from build123d import *

# Parameters (mm, degrees)
SKETCH1_R           = 12
SKETCH1_R_2         = 1.05
BOSS_EXTRUDE1_DEPTH = 9.1
HOLE2_D             = 7
HOLE2_DEPTH         = 12
HOLE2_CBORE_D       = 9
HOLE2_CBORE_DEPTH   = 3.9
SKETCH8_R           = 2.15
CUT_EXTRUDE1_DEPTH  = 6.2
FILLET1_R           = 1


with BuildPart() as part:
    # Sketch1 → Boss-Extrude1 (new body)
    with BuildSketch(Plane.XY):
        Circle(SKETCH1_R)
        with Locations((0, 8)):
            Circle(SKETCH1_R_2, mode=Mode.SUBTRACT)
        with Locations((8, 0)):
            Circle(SKETCH1_R_2, mode=Mode.SUBTRACT)
        with Locations((0, -8)):
            Circle(SKETCH1_R_2, mode=Mode.SUBTRACT)
    extrude(amount=BOSS_EXTRUDE1_DEPTH)

    # Hole2
    with Locations(Plane.XY.offset(9.1)):
        with Locations((-6, 0)):
            CounterBoreHole(HOLE2_D / 2, HOLE2_CBORE_D / 2, HOLE2_CBORE_DEPTH, depth=HOLE2_DEPTH)

    # Sketch8 → Cut-Extrude1 (cut)
    with BuildSketch(Plane(origin=(0, 0, 0), x_dir=(-1, 0, 0), z_dir=(0, 0, -1))):
        with Locations((0, 8)):
            Circle(SKETCH8_R)
        with Locations((0, -8)):
            Circle(SKETCH8_R)
        with Locations((-8, 0)):
            Circle(SKETCH8_R)
    extrude(amount=-CUT_EXTRUDE1_DEPTH, mode=Mode.SUBTRACT)

    # Fillet1
    fillet1_edges = [part.edges().sort_by_distance(p)[0] for p in [
        (-12, 0, 0),
        (-2.5, 0, 0),
        (-2.5, 0, 5.2),
        (-12, 0, 9.1),
    ]]
    fillet(fillet1_edges, radius=FILLET1_R - 0.0001)  # a hair under: the kernel refuses the full size


solid = part.part
Can you work these out from the model? Positions are in its coordinate system, mm. A direction names the side the tool comes from. Coordinates: 2 decimals unless noted, no trailing zeros. Order: outer loops, then holes, each group sorted by start corner. A loop starts at its lowest first (then second) coordinate and runs counter-clockwise, first axis right, second up. Notation, with made-up numbers: (84, 2) - (109, 2) arc R23 cw to (109, 31) - close; hole circle Ø11 at (4, 23.5). An arc over 180 degrees is marked (long way). Answer as a JSON object with one key per item and string values. Group by question number.
Q1. We'd pull the mould along X, two halves only. Please class faces 4 (the face through (-11.99, 0.53, 4.5)), 5 (the face through (0, 0, 0)), 6 (the face through (7, 1, 6.2)): +X half, -X half, draft (parallel to the pull), parting line (faces both ways), or undercut.
Q2. Imagine slicing it at B-B (x = 0). Please give me the cut outline in (y, z).
Q3. I need wall thicknesses on line 1 (Y direction, x = 0, z = 2.75); line 2 (Y direction, x = 0, z = 6.85); line 3 (X direction, y = -0.25, z = 2). Which ranges of each line are inside material? Lowest first, please. Write a range as from..to.
Q4. On a 3-axis mill with a long thin cutter (end or side, diameter ignored), from which of +Z, -Z, +X, -X, +Y, -Y can I reach the whole of each face in a straight line? I mean faces 1 (the face through (-10.496, 0.198, 7.177)), 2 (the face through (2, 0, 9.1)), 3 (the face through (-1, 9, 6.2)). Say none if no direction works.
Q5. Imagine slicing it at A-A (y = 0). Give the number of separate pieces and of enclosed holes in the cut face, and give its area (3 significant figures).
Q6. Will these pins go through, and if not, where does the flat tip stop? P1, Ø2, axis at x = 0.5, y = 7, coming from the -Z side; P2, Ø1.5, axis at x = -4.5, z = 2.5, coming from the +Y side; P3, Ø1.5, axis at x = 9, y = 8.5, coming from the +Z side.
Q7. Imagine slicing it at C-C (z = 2.5). Please give me the cut outline in (x, y).
Determined:
{
 "1": {"face 4": "parting line", "face 5": "draft", "face 6": "undercut"},
 "2": {"outline": "(-12, 1) arc R1 ccw to (-11, 0) - (-10.15, 0) - (-10.15, 6.2) - (-9.05, 6.2) - (-9.05, 9.1) - (-11, 9.1) arc R1 ccw to (-12, 8.1) - close; (-6.95, 6.2) - (-5.85, 6.2) - (-5.85, 0) - (5.85, 0) - (5.85, 6.2) - (6.95, 6.2) - (6.95, 9.1) - (-6.95, 9.1) - close; (9.05, 6.2) - (10.15, 6.2) - (10.15, 0) - (11, 0) arc R1 ccw to (12, 1) - (12, 8.1) arc R1 ccw to (11, 9.1) - (9.05, 9.1) - close"},
 "3": {"line 1": "y = -12..-10.15, -5.85..5.85, 10.15..12", "line 2": "y = -12..-9.05, -6.95..6.95, 9.05..12", "line 3": "x = -12..-9.49, -2.51..5.86, 10.14..12"},
 "4": {"face 1": "+Z", "face 2": "+Z, +X, -X, +Y, -Y", "face 3": "-Z"},
 "5": {"separate pieces": "3", "enclosed holes": "0", "area": "112 mm2"},
 "6": {"P1": "stops at z = 6.2", "P2": "stops at y = 11.4", "P3": "stops at z = 8.88"},
 "7": {"outline": "circle Ø24 at (0, 0); hole circle Ø7 at (-6, 0); hole circle Ø4.3 at (0, -8); hole circle Ø4.3 at (0, 8); hole circle Ø4.3 at (8, 0)"}
}
